from build123d import *

# Parameters (mm, degrees)
BOSS_EXTRUDE1_DEPTH = 3.175
SKETCH2_R           = 2.032
SKETCH2_R_2         = 1.5875
CUT_EXTRUDE1_DEPTH  = 40.767003046


with BuildPart() as part:
    # Sketch1 → Boss-Extrude1 (new body)
    with BuildSketch(Plane(origin=(0, 0, 0), x_dir=(0, 0, -1), z_dir=(1, 0, 0))):
        with BuildLine():
            Line((4.096045115, 32.429777905), (18.605696743, 7.969851937))
            ThreePointArc((18.605696743, 7.969851937), (18.535994972, 4.618026917), (15.499364997, 3.19729904))
            ThreePointArc((15.499364997, 3.19729904), (8.962719261, 2.075866472), (4.096045115, -2.429777905))
            ThreePointArc((4.096045115, -2.429777905), (-2.429777905, -4.096045115), (-4.096045115, 2.429777905))
            ThreePointArc((-4.096045115, 2.429777905), (-0.648204921, 15), (-4.096045115, 27.570222095))
            ThreePointArc((-4.096045115, 27.570222095), (-2.429777905, 34.096045115), (4.096045115, 32.429777905))
        make_face()
    extrude(amount=BOSS_EXTRUDE1_DEPTH)

    # Sketch2 → Cut-Extrude1 (cut, through all)
    with BuildSketch(Plane(origin=(3.175, 0, 0), x_dir=(0, 0, -1), z_dir=(1, 0, 0))):
        with Locations((0, 30)):
            Circle(SKETCH2_R)
        Circle(SKETCH2_R)
        with Locations((15.875, 6.35)):
            Circle(SKETCH2_R_2)
    extrude(amount=-CUT_EXTRUDE1_DEPTH, mode=Mode.SUBTRACT)


solid = part.part
Work out the finished part from the listing and answer in its coordinate system (mm). Round coordinates to 2 decimals unless told otherwise and drop trailing zeros. Write each loop counter-clockwise with the first axis right and the second up, starting at its lowest first coordinate (ties: lowest second). Pieces come first, ordered by that corner, then holes.
1) Straight lines are drawn through the part: line 1 (Y direction, x = 2.35, z = 0); line 2 (Y direction, x = 2.15, z = -16); line 3 (Z direction, x = 1.9, y = 30.5). For each, find the intervals that lie inside material, in ascending order.
2) A cutting plane is placed at D-D (y = 30). Give the vertices of the cut face in (x, z) (1 decimal).
3) A cutting plane is placed at B-B (y = 0). Give the vertices of the cut face in (x, z) (1 decimal), plus the area to 3 significant figures.
4) A cutting plane is placed at C-C (x = 0.4). Give the number of separate pieces and of enclosed holes in the cut face, plus the area to 3 significant figures.
5) The mould has two halves that part along Z. Classify faces 1 (the flat face through (0, 15, -5)), 2 (the cylindrical face through (1.57, -4.15, 2.34)), 3 (the cylindrical face through (1.57, 2.12, -9.05)): pulls with the +Z half, pulls with the -Z half, needs draft (parallel to the pull), parting line crosses it, or undercut.
6) A cutting plane is placed at A-A (z = 0). Give the vertices of the cut face in (x, y) (1 decimal).
7) Given pin 1 Ø3.5 at (y, z) = (30, 0) entering from +X; pin 2 Ø1.5 at (x, y) = (2.5, 16) entering from +Z, each flat-ended and moving along its own axis, determine where each tip first touches the part or whether it passes through.
Completed:
1. line 1: y = -4.76 to -2.03, 2.03 to 27.97, 32.03 to 34.76
1. line 2: y = 3.18 to 4.77, 7.93 to 12.36
1. line 3: z = -5.24 to -1.97, 1.97 to 4.74
2. outline: (0, -5.5) - (3.2, -5.5) - (3.2, -2) - (0, -2) - close; (0, 2) - (3.2, 2) - (3.2, 4.8) - (0, 4.8) - close
3. outline: (0, -6) - (3.2, -6) - (3.2, -2) - (0, -2) - close; (0, 2) - (3.2, 2) - (3.2, 4.8) - (0, 4.8) - close
3. area: 21.3 mm2
4. separate pieces: 1
4. enclosed holes: 3
4. area: 487 mm2
5. face 1: needs draft
5. face 2: parting line crosses it
5. face 3: undercut
6. outline: (0, -4.8) - (3.2, -4.8) - (3.2, -2) - (0, -2) - close; (0, 2) - (3.2, 2) - (3.2, 28) - (0, 28) - close; (0, 32) - (3.2, 32) - (3.2, 34.8) - (0, 34.8) - close
7. pin 1: passes through
7. pin 2: stops at z = 0.71
